Input: part model. Units: mm. Frame: model coordinates. A direction names the side the tool comes from. Give positions to 0.01 mm unless a question says otherwise; leave off trailing zeros. Loops run counter-clockwise (first coordinate to the right, second up) from the corner with the lowest first, then second, coordinate; pieces in that order, holes last. Notation, with made-up numbers: (-32, 62.25) - (-22, 62.25) arc R17 cw to (-22, 66.25) - close; hole circle Ø3 at (-19, 48). An arc over 180 degrees is marked (long way). Answer as a JSON object with one key per item and string values.
from build123d import *

# Parameters (mm, degrees)
SKETCH3_R          = 2
CUT_EXTRUDE1_DEPTH = 14.8
CUT_EXTRUDE2_START = -2
SKETCH4_R          = 5
CUT_EXTRUDE2_DEPTH = 12.8


with BuildPart() as part:
    # Sketch2 → Revolve1 (revolve)
    with BuildSketch(Plane(origin=(0, 0, 0), x_dir=(1, 0, 0), z_dir=(0, 1, 0))):
        Polygon((-7.7, 12), (-7.7, 0), (-7.1, 0), (7.1, 0), (7.1, 12), (6.6, 12), (4.6, 10), (-4.6, 10), (-6.6, 12), (-7.1, 12), align=None)
    revolve(axis=Axis((7.1, 0, 0), (-1, 0, 0)))

    # Sketch3 → Cut-Extrude1 (cut)
    with BuildSketch(Plane.ZY.offset(7.7)):
        Circle(SKETCH3_R)
    extrude(amount=-CUT_EXTRUDE1_DEPTH, mode=Mode.SUBTRACT)

    # Sketch4 → Cut-Extrude2 (cut)
    with BuildSketch(Plane.ZY.offset(7.7).offset(CUT_EXTRUDE2_START)):
        Circle(SKETCH4_R)
    extrude(amount=-CUT_EXTRUDE2_DEPTH, mode=Mode.SUBTRACT)


solid = part.part
Item 1: Access query for faces 4 (the face through (-0.06, 9.76, 2.17)), 5 (the face through (6.85, -0.53, 11.99)), 6 (the face through (-5.7, -2.2, -0.1)). Directions: +Z, -Z, +X, -X, +Y, -Y. A direction counts if a zero-diameter tool reaches every point of the face in a straight line with its end or side. Return the directions, or none.
Geometry check:
{"face 4": "none", "face 5": "+X, -X", "face 6": "+X"}
Item 2: Cut plane A-A (z = 0). Return loops of the section in (x, y).
Geometry check:
{"outline": "(-7.7, -12) - (-6.6, -12) - (-4.6, -10) - (4.6, -10) - (6.6, -12) - (7.1, -12) - (7.1, -5) - (-5.7, -5) - (-5.7, -2) - (-7.7, -2) - close; (-7.7, 2) - (-5.7, 2) - (-5.7, 5) - (7.1, 5) - (7.1, 12) - (6.6, 12) - (4.6, 10) - (-4.6, 10) - (-6.6, 12) - (-7.7, 12) - close"}
Item 3: Contact query for flat-ended pins moving along their axis: P1, Ø1.5, axis at x = -5, z = 5, coming from the +Y side; P2, Ø6.5, axis at y = 0, z = 0, coming from the -X side; P3, Ø6, axis at x = 0.5, y = 3.5, coming from the +Z side; P4, Ø3, axis at x = -2.5, y = 9.5, coming from the +Z side. Output: stop coordinate, or through.
Geometry check:
{"P1": "stops at y = 10.04", "P2": "stops at x = -7.7", "P3": "stops at z = 9.99", "P4": "stops at z = 6"}
Item 4: Mould query, pull axis Z, two halves, no side actions, for faces 1 (the face through (0.61, -4.88, -1.08)), 2 (the face through (-4.725, 9.884, 2.195)), 3 (the face through (7.1, -0.2, 5.2)). Classes: released by +Z, released by -Z, zero draft, split by the parting line, or undercut.
Geometry check:
{"face 1": "undercut", "face 2": "split by the parting line", "face 3": "zero draft"}
Item 5: Cut plane C-C (x = 4). Return loops of the section in (y, z).
Geometry check:
{"outline": "circle Ø20 at (0, 0); hole circle Ø10 at (0, 0)"}
Item 6: Material intervals for line 1 (Y direction, x = 4.25, z = 0); line 2 (Z direction, x = 2.75, y = 0.5); line 3 (X direction, y = -1.75, z = 2), sorted ascending. Write a range as [from, to].
Geometry check:
{"line 1": "y = [-10, -5], [5, 10]", "line 2": "z = [-9.99, -4.97], [4.97, 9.99]", "line 3": "x = [-7.7, -5.7]"}
